Part model, mm, in its own coordinate system. A direction names the side the tool comes from. Round coordinates to 2 decimals unless told otherwise and drop trailing zeros. Loops run counter-clockwise (first coordinate to the right, second up) from the corner with the lowest first, then second, coordinate; pieces in that order, holes last. Notation, with made-up numbers: M -21.75,45 L 35.25,45 A9 ccw 35.25,54 Z; hole C -4.5,32 d8. An arc over 180 degrees is marked long. Put each result on its own line as item: value. Start each with the question number.
1) Drop flat-ended pins along their axis: pin 1 Ø6 at (y, z) = (-26, -3) entering from -X; pin 2 Ø1.5 at (y, z) = (7, 2) entering from -X. Give the stop position or say it passes through.
2) Slice it at C-C on y = -39. Give the cut face in (x, z).
3) Which spindle directions (+Z, -Z, +X, -X, +Y, -Y) get a long thin tool onto all of the face, cutting with end or side? Do faces 4 (the flat face through (0, -16, 3)), 5 (the flat face through (-5.22, 10.6, 2.96)), 6 (the cylindrical face through (0.13, 18.542, -4.914)), 7 (the cylindrical face through (-1.156, 25.05, 0.392)), 8 (the flat face through (0, 28.7, 2)). Say none if no direction does.
4) Probe line 1 along Y through (x, z) = (-2.75, 5); line 2 along Y through (x, z) = (3.5, -4.5); line 3 along Z through (x, y) = (0.25, -43). List the from-to ranges inside material, lowest first.
5) Slice it at B-B on z = 1.9. Give the cut face in (x, y), then the cut area to 3 significant figures.
6) Slice it at D-D on y = -5.5. Give the cut face in (x, z), then the cut area to 3 significant figures.
7) Slice it at A-A on x = 0. Give the cut face in (y, z), then the cut area to 3 significant figures.
8) Pull direction X, two halves, no side cores. Call faces 1 (the flat face through (5.172, 10.599, 3.042)), 2 (the flat face through (0, -16, 2)), 3 (the flat face through (0, 15.5, -5.2)): +X half, -X half, draft (parallel to the pull), parting line (faces both ways), or undercut.
```python
from build123d import *

# Parameters (mm, degrees)
BOSS_EXTRUDE1_DEPTH = 21.5
SKETCH2_R           = 1.9
BOSS_EXTRUDE2_DEPTH = 7.2
CUT_EXTRUDE1_DEPTH  = 6
BOSS_EXTRUDE3_START = 16
SKETCH4_R           = 1.9
BOSS_EXTRUDE3_DEPTH = 16
SKETCH5_R           = 0.8
SKETCH5_R_2         = 0.654757234
BOSS_EXTRUDE4_DEPTH = 34.5


with BuildPart() as part:
    # Sketch1 → Boss-Extrude1 (new body)
    with BuildSketch(Plane(origin=(0, 0, 0), x_dir=(1, 0, 0), z_dir=(0, 1, 0))):
        Polygon((-6.92820323, 0), (-3.464101615, -6), (3.464101615, -6), (6.92820323, 0), (3.464101615, 6), (-3.464101615, 6), align=None)
    extrude(amount=BOSS_EXTRUDE1_DEPTH)

    # Sketch2 → Boss-Extrude2 (add)
    with BuildSketch(Plane(origin=(0, 21.5, 0), x_dir=(1, 0, 0), z_dir=(0, 1, 0))):
        with Locations(Location((0, -1.9, 0), (0, 0, 270))):
            Circle(SKETCH2_R)
    extrude(amount=BOSS_EXTRUDE2_DEPTH)

    # Sketch3 → Cut-Extrude1 (cut)
    with BuildSketch(Plane(origin=(0, 21.5, 0), x_dir=(1, 0, 0), z_dir=(0, 1, 0))):
        with BuildLine():
            Line((-6.661546125, -0.461863655), (-6.92820323, 0))
            Line((-6.92820323, 0), (-3.464101615, 6))
            Line((-3.464101615, 6), (3.464101615, 6))
            Line((3.464101615, 6), (6.92820323, 0))
            Line((6.92820323, 0), (6.661546125, -0.461863655))
            ThreePointArc((6.661546125, -0.461863655), (0, 4.915015255), (-6.661546125, -0.461863655))
        make_face()
    extrude(amount=-CUT_EXTRUDE1_DEPTH, mode=Mode.SUBTRACT)

    # Sketch4 → Boss-Extrude3 (add)
    with BuildSketch(Plane.XZ.offset(BOSS_EXTRUDE3_START)):
        with Locations(Location((0, 1.9, 0), (0, 0, 90))):
            Circle(SKETCH4_R)
    extrude(amount=-BOSS_EXTRUDE3_DEPTH)

    # Sketch5 → Boss-Extrude4 (add)
    with BuildSketch(Plane.XZ.offset(16)):
        with Locations(Location((0, 1.9, 0), (0, 0, 270))):
            Circle(SKETCH5_R)
        with Locations(Location((0, 1.9, 0), (0, 0, 270))):
            Circle(SKETCH5_R_2, mode=Mode.SUBTRACT)
    extrude(amount=BOSS_EXTRUDE4_DEPTH)


solid = part.part
```
Recorded:
1. pin 1: passes through
1. pin 2: stops at x = -6.21
2. outline: C 0,1.9 d1.6; hole C 0,1.9 d1.31
3. face 4: -Y
3. face 5: +Z, -X, +Y, -Y
3. face 6: -Z, +Y
3. face 7: +Y
3. face 8: +Z, -Z, +X, -X, +Y
4. line 1: y = 0 to 21.5
4. line 2: y = 0 to 15.5
4. line 3: z = 1.14 to 1.29, 2.51 to 2.66
5. outline: M -5.83,0 L -1.9,0 L -1.9,-16 L -0.8,-16 L -0.8,-50.5 L -0.65,-50.5 L -0.65,-16 L 0.65,-16 L 0.65,-50.5 L 0.8,-50.5 L 0.8,-16 L 1.9,-16 L 1.9,0 L 5.83,0 L 5.83,21.5 L 1.9,21.5 L 1.9,28.7 L -1.9,28.7 L -1.9,21.5 L -5.83,21.5 Z
5. area: 349 mm2
6. outline: C 0,1.9 d3.8
6. area: 11.3 mm2
7. outline: M -50.5,1.1 L -16,1.1 L -16,0 L 0,0 L 0,-6 L 15.5,-6 L 15.5,-4.92 L 21.5,-4.92 L 21.5,0 L 28.7,0 L 28.7,3.8 L 21.5,3.8 L 21.5,6 L 0,6 L 0,3.8 L -16,3.8 L -16,2.7 L -50.5,2.7 L -50.5,2.55 L -16,2.55 L -16,1.25 L -50.5,1.25 Z
7. area: 350 mm2
8. face 1: +X half
8. face 2: undercut
8. face 3: draft
